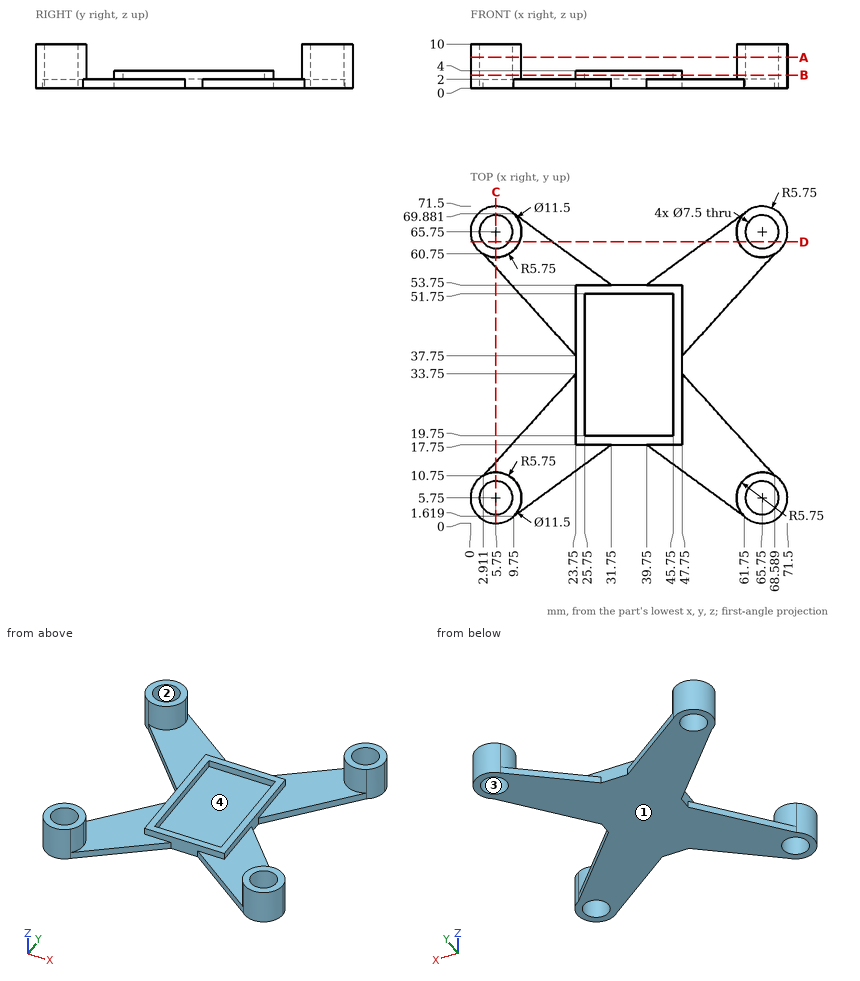
Here's the drawing with two shaded views (mm, measured from the low corner). I have some questions. A direction names the side the tool comes from. Give positions to 0.01 mm unless a question says otherwise; leave off trailing zeros. Order: outer loops, then holes, each group sorted by start corner. A loop starts at its lowest first (then second) coordinate and runs counter-clockwise, first axis right, second up. Notation, with made-up numbers: M -26,16.25 L -8,16.25 A17 ccw -8,20.25 Z; hole C 10.25,71.25 d9. An arc over 180 degrees is marked long. Answer as a JSON object with one key per item and string values. Group by question number.
1) On a 3-axis mill with a long thin cutter (end or side, diameter ignored), from which of +Z, -Z, +X, -X, +Y, -Y can I reach the whole of each face in a straight line? I mean the marked faces 3 and 4. Say none if no direction works.
2) Suppose I cut it at A-A, the plane z = 7. Write out the boundary of the cut face in (x, y).
3) Suppose I cut it at B-B, the plane z = 3. Count the separate pieces of the cut face and the enclosed holes in it.
4) Suppose I cut it at C-C, the plane x = 5.75. Write out the boundary of the cut face in (y, z).
5) Suppose I cut it at D-D, the plane y = 63.5. Write out the boundary of the cut face in (x, z), plus the area to 3 significant figures.
6) Please list where these lines run through material, in increasing order: L1, parallel to Y at x = 65.75, z = 7.5; L2, parallel to X at y = 64.5, z = 1 (1 decimal); L3, parallel to X at y = 48.5, z = 3.25. Write a range as [from, to].
7) We'd pull the mould along X, two halves only. Please class the marked faces 1 and 2: pulls with the +X half, pulls with the -X half, needs draft (parallel to the pull), parting line crosses it, or undercut.
8) I'm going to push flat-ended pins straight in: pin 1 Ø8.5 at (x, y) = (13.5, 11.5) entering from +Z; pin 2 Ø1.6 at (y, z) = (40, 3) entering from -X; pin 3 Ø4.5 at (x, y) = (5.75, 65.75) entering from +Z; pin 4 Ø2 at (x, z) = (35.5, 2) entering from +Y. Where does each tip first touch, or does it pass through?
Results found:
{
 "1": {"face 3": "+Z, -Z", "face 4": "+Z"},
 "2": {"outline": "M 9.75,1.62 A5.75 ccw 11.5,5.75 A5.75 ccw long Z; M 9.75,69.88 A5.75 ccw long 11.5,65.75 A5.75 ccw Z; M 68.59,10.75 A5.75 ccw long 71.5,5.75 A5.75 ccw Z; M 68.59,60.75 A5.75 ccw 71.5,65.75 A5.75 ccw long Z; hole C 5.75,5.75 d7.5; hole C 5.75,65.75 d7.5; hole C 65.75,5.75 d7.5; hole C 65.75,65.75 d7.5"},
 "3": {"separate pieces": "5", "enclosed holes": "5"},
 "4": {"outline": "M 0,0 L 2,0 L 2,10 L 0,10 Z; M 9.5,0 L 13.88,0 L 13.88,2 L 11.5,2 L 11.5,10 L 9.5,10 Z; M 57.62,0 L 62,0 L 62,10 L 60,10 L 60,2 L 57.62,2 Z; M 69.5,0 L 71.5,0 L 71.5,10 L 69.5,10 Z"},
 "5": {"outline": "M 0.46,0 L 2.75,0 L 2.75,10 L 0.46,10 Z; M 8.75,0 L 18.45,0 L 18.45,2 L 11.04,2 L 11.04,10 L 8.75,10 Z; M 53.05,0 L 62.75,0 L 62.75,10 L 60.46,10 L 60.46,2 L 53.05,2 Z; M 68.75,0 L 71.04,0 L 71.04,10 L 68.75,10 Z", "area": "121 mm²"},
 "6": {"L1": "[0, 2], [9.5, 11.5], [60, 62], [69.5, 71.5]", "L2": "[0.1, 2.2], [9.3, 17.1], [54.4, 62.2], [69.3, 71.4]", "L3": "[23.75, 25.75], [45.75, 47.75]"},
 "7": {"face 1": "needs draft", "face 2": "undercut"},
 "8": {"pin 1": "z = 10", "pin 2": "x = 23.75", "pin 3": "through", "pin 4": "y = 53.75"}
}
